Part model, mm, in its own coordinate system. A direction names the side the tool comes from. Give positions to 0.01 mm unless a question says otherwise; leave off trailing zeros. Order: outer loops, then holes, each group sorted by start corner. A loop starts at its lowest first (then second) coordinate and runs counter-clockwise, first axis right, second up. Notation, with made-up numbers: (-31, -6.5) - (2, -6.5) arc R29 ccw to (2, 18.5) - close; hole circle Ø2 at (59.25, 65). An arc over 180 degrees is marked (long way). One line per item, written item: value.
```python
from build123d import *

# Parameters (mm, degrees)
SKETCH1_W           = 6.096
SKETCH1_H           = 6.096
BOSS_EXTRUDE1_DEPTH = 5.08
SKETCH2_W           = 7.62
SKETCH2_H           = 7.62
BOSS_EXTRUDE2_DEPTH = 5.08
FILLET1_R           = 2.54
FILLET2_R           = 2.54
SKETCH4_W           = 7.62
SKETCH4_H           = 5.08
BOSS_EXTRUDE4_DEPTH = 31.75
SKETCH5_W           = 3.81
SKETCH5_H           = 39.37
CUT_EXTRUDE1_DEPTH  = 2.54
SKETCH7_W           = 7.62
SKETCH7_H           = 2.54
BOSS_EXTRUDE5_DEPTH = 19.05


with BuildPart() as part:
    # Sketch1 → Boss-Extrude1 (new body)
    with BuildSketch(Plane(origin=(0, 0, 0), x_dir=(1, 0, 0), z_dir=(0, 1, 0))):
        with Locations((3.048, 3.048)):
            Rectangle(SKETCH1_W, SKETCH1_H)
    extrude(amount=BOSS_EXTRUDE1_DEPTH)

    # Sketch2 → Boss-Extrude2 (add)
    with BuildSketch(Plane(origin=(0, 5.08, 0), x_dir=(1, 0, 0), z_dir=(0, 1, 0))):
        with Locations((3.048, 3.048)):
            Rectangle(SKETCH2_W, SKETCH2_H)
    extrude(amount=BOSS_EXTRUDE2_DEPTH)

    # Fillet1
    # the kernel refuses this fillet: 2.54 mm, written as the material it adds along each edge
    with BuildSketch(Plane(origin=(0, 5.08, -6.096), x_dir=(-1, 0, 0), z_dir=(0, 0, 1))) as fillet1_piece_1:
        with BuildLine():
            CenterArc((2.54, 1.813922821), FILLET1_R, 180, 45.572995999)
            Line((0, 1.813922821), (-0.0508, 1.813922821))
            Line((-0.0508, 1.813922821), (-0.0508, 0))
            Line((-0.0508, 0), (0, -0.0508))
            ThreePointArc((0, -0.0508), (0.381, -0.0508), (0.72644, -0.036278456))
            Line((0.72644, -0.036278456), (0.762, 0))
        make_face()
    extrude(amount=6.096)

    # Fillet2
    # the kernel refuses this fillet: 2.54 mm, written as the material it adds along each edge
    with BuildSketch(Plane(origin=(6.096, 5.08, 0), x_dir=(0, -1, 0), z_dir=(-1, 0, 0))) as fillet2_piece_1_section:
        with BuildLine():
            CenterArc((1.813922821, 2.54), FILLET2_R, 224.427004001, 45.572995999)
            Line((0, 0.762), (-0.036278456, 0.72644))
            ThreePointArc((-0.036278456, 0.72644), (-0.0508, 0.381), (-0.0508, 0))
            Line((-0.0508, 0), (0, -0.0508))
            Line((0, -0.0508), (1.813922821, -0.0508))
            Line((1.813922821, -0.0508), (1.813922821, 0))
        make_face()
    fillet2_piece_1 = extrude(amount=6.858, mode=Mode.PRIVATE)
    fillet2_piece_1 = fillet2_piece_1 - Plane(origin=(-2.54, 3.266077179, 0.188412047), x_dir=(-1, 0, 0), z_dir=(0, 0, -1)) * Cylinder(2.54, 21, mode=Mode.PRIVATE)
    add(fillet2_piece_1)
    with BuildSketch(Plane(origin=(6.096, 5.08, 0), x_dir=(0, -1, 0), z_dir=(0, 0, -1))) as fillet2_piece_2:
        with BuildLine():
            CenterArc((1.813922821, -2.54), FILLET2_R, 90, 45.572995999)
            Line((0, -0.762), (-0.036278456, -0.72644))
            ThreePointArc((-0.036278456, -0.72644), (-0.0508, -0.381), (-0.0508, 0))
            Line((-0.0508, 0), (0, 0.0508))
            Line((0, 0.0508), (1.813922821, 0.0508))
            Line((1.813922821, 0.0508), (1.813922821, 0))
        make_face()
    extrude(amount=6.096)
    with BuildSketch(Plane(origin=(-0.762, 5.08, -6.096), x_dir=(0, 0, -1), z_dir=(1, 0, 0))) as fillet2_piece_3_section:
        with BuildLine():
            CenterArc((2.54, -1.813922821), FILLET2_R, 134.427004001, 45.572995999)
            Line((0, -1.813922821), (-0.0508, -1.813922821))
            Line((-0.0508, -1.813922821), (-0.0508, 0))
            Line((-0.0508, 0), (0, 0.0508))
            ThreePointArc((0, 0.0508), (0.381, 0.0508), (0.72644, 0.036278456))
            Line((0.72644, 0.036278456), (0.762, 0))
        make_face()
    fillet2_piece_3 = extrude(amount=6.858, mode=Mode.PRIVATE)
    fillet2_piece_3 = fillet2_piece_3 - Plane(origin=(-2.54, 3.266077179, -6.345051063), x_dir=(-1, 0, 0), z_dir=(0, 0, -1)) * Cylinder(2.54, 21, mode=Mode.PRIVATE)
    add(fillet2_piece_3)
    with BuildSketch(Plane(origin=(10.630807052, 5.08, 0), x_dir=(0, -1, 0), z_dir=(-1, 0, 0))) as fillet2_piece_4a_section:
        with BuildLine():
            CenterArc((1.813922821, 2.54), FILLET2_R, 224.427004001, 45.572995999)
            Line((0, 0.762), (-0.036278456, 0.72644))
            ThreePointArc((-0.036278456, 0.72644), (-0.0508, 0.381), (-0.0508, 0))
            Line((-0.0508, 0), (0, -0.0508))
            Line((0, -0.0508), (1.813922821, -0.0508))
            Line((1.813922821, -0.0508), (1.813922821, 0))
        make_face()
    fillet2_piece_4a = extrude(amount=11.392807052, mode=Mode.PRIVATE)
    fillet2_piece_4a = split(fillet2_piece_4a, bisect_by=Plane(origin=(6.096, 4.594869389, 0.188412047), z_dir=(1, 0, 0)), keep=Keep.TOP, mode=Mode.PRIVATE)
    fillet2_piece_4a = split(fillet2_piece_4a, bisect_by=Plane(origin=(6.858, 4.594869389, 0.188412047), z_dir=(-1, 0, 0)), keep=Keep.TOP, mode=Mode.PRIVATE)
    with BuildSketch(Plane(origin=(6.096, 5.08, 4.534807052), x_dir=(0, -1, 0), z_dir=(0, 0, -1))) as fillet2_piece_4b_section:
        with BuildLine():
            CenterArc((1.813922821, -2.54), FILLET2_R, 90, 45.572995999)
            Line((0, -0.762), (-0.036278456, -0.72644))
            ThreePointArc((-0.036278456, -0.72644), (-0.0508, -0.381), (-0.0508, 0))
            Line((-0.0508, 0), (0, 0.0508))
            Line((0, 0.0508), (1.813922821, 0.0508))
            Line((1.813922821, 0.0508), (1.813922821, 0))
        make_face()
    fillet2_piece_4b = extrude(amount=10.630807052, mode=Mode.PRIVATE)
    fillet2_piece_4b = split(fillet2_piece_4b, bisect_by=Plane(origin=(6.284412047, 4.594869389, 0), z_dir=(0, 0, 1)), keep=Keep.TOP, mode=Mode.PRIVATE)
    fillet2_piece_4b = split(fillet2_piece_4b, bisect_by=Plane(origin=(6.284412047, 4.594869389, 0.762), z_dir=(0, 0, -1)), keep=Keep.TOP, mode=Mode.PRIVATE)
    fillet2_piece_4 = fillet2_piece_4a & fillet2_piece_4b
    add(fillet2_piece_4)
    with BuildSketch(Plane(origin=(6.096, 5.08, 0), x_dir=(0, -1, 0), z_dir=(0, 0, -1))) as fillet2_piece_5a_section:
        with BuildLine():
            CenterArc((1.813922821, -2.54), FILLET2_R, 90, 45.572995999)
            Line((0, -0.762), (-0.036278456, -0.72644))
            ThreePointArc((-0.036278456, -0.72644), (-0.0508, -0.381), (-0.0508, 0))
            Line((-0.0508, 0), (0, 0.0508))
            Line((0, 0.0508), (1.813922821, 0.0508))
            Line((1.813922821, 0.0508), (1.813922821, 0))
        make_face()
    fillet2_piece_5a = extrude(amount=10.630807052, mode=Mode.PRIVATE)
    fillet2_piece_5a = split(fillet2_piece_5a, bisect_by=Plane(origin=(6.284412047, 4.594869389, -6.096), z_dir=(0, 0, -1)), keep=Keep.TOP, mode=Mode.PRIVATE)
    fillet2_piece_5a = split(fillet2_piece_5a, bisect_by=Plane(origin=(6.284412047, 4.594869389, -6.858), z_dir=(0, 0, 1)), keep=Keep.TOP, mode=Mode.PRIVATE)
    with BuildSketch(Plane(origin=(-0.762, 5.08, -6.096), x_dir=(0, 0, -1), z_dir=(1, 0, 0))) as fillet2_piece_5b_section:
        with BuildLine():
            CenterArc((2.54, -1.813922821), FILLET2_R, 134.427004001, 45.572995999)
            Line((0, -1.813922821), (-0.0508, -1.813922821))
            Line((-0.0508, -1.813922821), (-0.0508, 0))
            Line((-0.0508, 0), (0, 0.0508))
            ThreePointArc((0, 0.0508), (0.381, 0.0508), (0.72644, 0.036278456))
            Line((0.72644, 0.036278456), (0.762, 0))
        make_face()
    fillet2_piece_5b = extrude(amount=11.392807052, mode=Mode.PRIVATE)
    fillet2_piece_5b = split(fillet2_piece_5b, bisect_by=Plane(origin=(6.096, 4.594869389, -6.284412047), z_dir=(1, 0, 0)), keep=Keep.TOP, mode=Mode.PRIVATE)
    fillet2_piece_5b = split(fillet2_piece_5b, bisect_by=Plane(origin=(6.858, 4.594869389, -6.284412047), z_dir=(-1, 0, 0)), keep=Keep.TOP, mode=Mode.PRIVATE)
    fillet2_piece_5 = fillet2_piece_5a & fillet2_piece_5b
    add(fillet2_piece_5)

    # Sketch4 → Boss-Extrude4 (add)
    with BuildSketch(Plane(origin=(0, 0, -6.858), x_dir=(-1, 0, 0), z_dir=(0, 0, -1))):
        with Locations((-3.048, 7.62)):
            Rectangle(SKETCH4_W, SKETCH4_H)
    extrude(amount=BOSS_EXTRUDE4_DEPTH)

    # Sketch5 → Cut-Extrude1 (cut)
    with BuildSketch(Plane(origin=(0, 10.16, 0), x_dir=(1, 0, 0), z_dir=(0, 1, 0))):
        with Locations((3.048, 18.923)):
            Rectangle(SKETCH5_W, SKETCH5_H)
    extrude(amount=-CUT_EXTRUDE1_DEPTH, mode=Mode.SUBTRACT)

    # Sketch7 → Boss-Extrude5 (add)
    with BuildSketch(Plane.XZ.offset(-5.08)):
        with Locations((3.048, -37.338)):
            Rectangle(SKETCH7_W, SKETCH7_H)
    extrude(amount=BOSS_EXTRUDE5_DEPTH)


solid = part.part
```
1) Slice it at B-B on x = 4.5. Write the cut outline in (y, z), then the cut area to 3 significant figures.
Answer:
outline: (-13.97, -38.61) - (7.62, -38.61) - (7.62, 0.76) - (5.08, 0.76) arc R2.54 cw to (3.27, 0) - (0, 0) - (0, -6.1) - (3.27, -6.1) arc R2.54 cw to (5.08, -6.86) - (5.08, -36.07) - (-13.97, -36.07) - close
area: 180 mm2
2) Which spindle directions (+Z, -Z, +X, -X, +Y, -Y) get a long thin tool onto all of the face, cutting with end or side? Do faces 5 (the face through (-0.204, 4.263, -3.101)), 6 (the face through (6, 10.16, -19)), 7 (the face through (3, 7.62, -19)), 8 (the face through (3, 2, -6.096)), 9 (the face through (3, 0, -3)). Say none if no direction does.
Answer:
face 5: +Z, -X, -Y
face 6: +Z, -Z, +X, -X, +Y
face 7: +Z, -Z, +Y
face 8: +X, -X, -Y
face 9: +Z, +X, -X, -Y
3) Slice it at C-C on z = -35. Write the cut outline in (x, y), then the cut area to 3 significant figures.
Answer:
outline: (-0.76, 5.08) - (6.86, 5.08) - (6.86, 10.16) - (4.95, 10.16) - (4.95, 7.62) - (1.14, 7.62) - (1.14, 10.16) - (-0.76, 10.16) - close
area: 29.0 mm2
4) Slice it at A-A on y = 1.5. Write the cut outline in (x, z).
Answer:
outline: (-0.76, -38.61) - (6.86, -38.61) - (6.86, -36.07) - (-0.76, -36.07) - close; (0, -6.1) - (6.1, -6.1) - (6.1, 0) - (0, 0) - close
5) Slice it at D-D on y = 8.5. Write the cut outline in (x, z).
Answer:
outline: (-0.76, -38.61) - (1.14, -38.61) - (1.14, 0.76) - (-0.76, 0.76) - close; (4.95, -38.61) - (6.86, -38.61) - (6.86, 0.76) - (4.95, 0.76) - close
6) Drop flat-ended pins along their axis: P1, Ø1, axis at y = 2, z = -3, coming from the -X side; P2, Ø1.1, axis at x = 2.5, z = -27.5, coming from the +Y side; P3, Ø3, axis at x = 1.5, z = -9, coming from the -Y side. Give the stop position or say it passes through.
Answer:
P1: stops at x = 0
P2: stops at y = 7.62
P3: stops at y = 5.08
7) Wall check: line 1 along Z through (x, y) = (6, 3); line 2 along Z through (x, y) = (1.75, -7.5); line 3 along Y through (x, z) = (1, -23). Give the ranges that are in metal, low to high. Write a range as [from, to].
Answer:
line 1: z = [-38.61, -36.07], [-6.1, 0]
line 2: z = [-38.61, -36.07]
line 3: y = [5.08, 10.16]
8) Two-plate mould, pull along Z, no slides. Class faces 1 (the face through (6.096, 2, -3)), 2 (the face through (3, 5.08, -21)), 3 (the face through (3, -2, -38.608)), 4 (the face through (3, 7, 0.762)): pulls with the +Z half, pulls with the -Z half, needs draft (parallel to the pull), parting line crosses it, or undercut.
Answer:
face 1: needs draft
face 2: undercut
face 3: pulls with the -Z half
face 4: pulls with the +Z half
